Design review of the part shown in the three views and the two pictorial views. Dimensions are in mm from the part's minimum x, y and z. Give positions to 0.01 mm unless a question says otherwise; leave off trailing zeros. Order: outer loops, then holes, each group sorted by start corner. A loop starts at its lowest first (then second) coordinate and runs counter-clockwise, first axis right, second up. Notation, with made-up numbers: (81.25, 63) - (94.25, 63) arc R34 ccw to (94.25, 102) - close; hole circle Ø6 at (-32.5, 68.5). An arc over 180 degrees is marked (long way). Put each result on its own line as item: value.
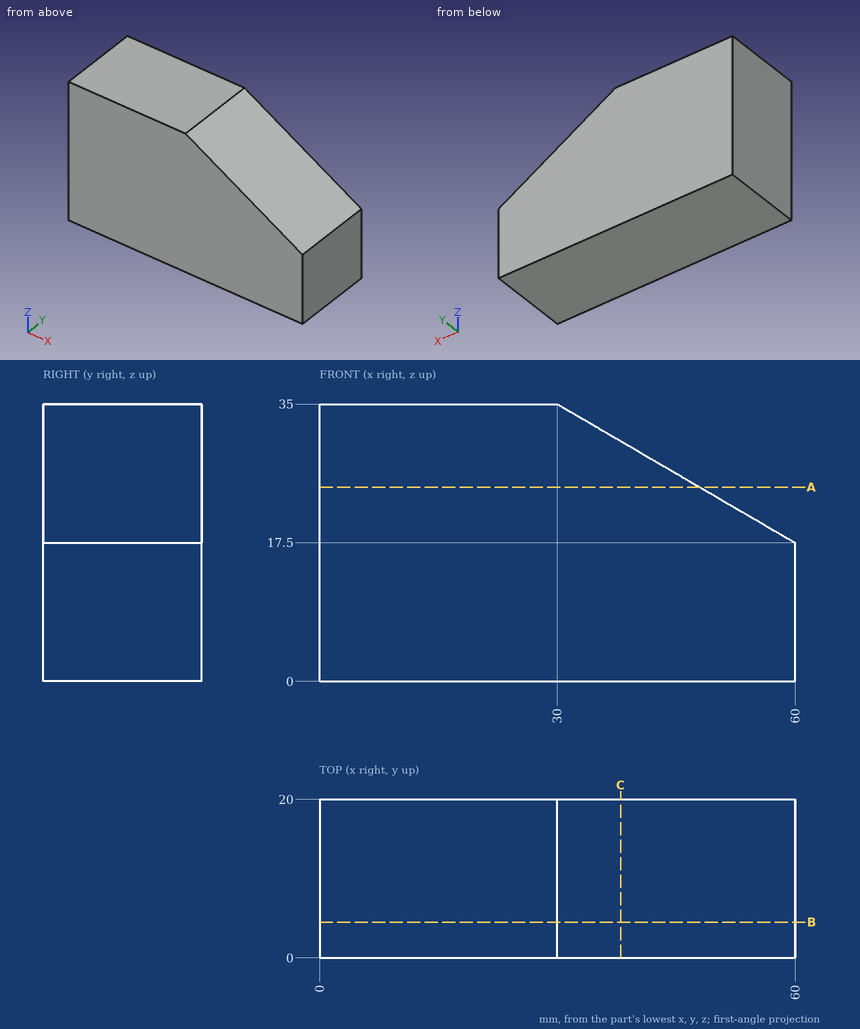
(1) Take a section at C-C, the plane x = 38. Write out the cut boundary in (y, z), then the cut area to 3 significant figures.
The answers:
outline: (0, 0) - (20, 0) - (20, 30.33) - (0, 30.33) - close
area: 607 mm^2
(2) Take a section at B-B, the plane y = 4.5. Write out the cut boundary in (x, z), then the cut area to 3 significant figures.
The answers:
outline: (0, 0) - (60, 0) - (60, 17.5) - (30, 35) - (0, 35) - close
area: 1,840 mm^2
(3) Clearance check with a flat-ended pin moving along its axis: pin 1 Ø4 at (y, z) = (17.5, 20) entering from +X. State where the tip first meets the part, or that it passes through.
The answers:
pin 1: x = 59.14
(4) Wall thickness on L1, parallel to X at y = 4.5, z = 18; L2, parallel to X at y = 5.5, z = 22.5; L3, parallel to Z at x = 43, y = 3: over which ranges is each line inside the solid? List them lowest first.
The answers:
L1: 0 to 59.14
L2: 0 to 51.43
L3: 0 to 27.42
(5) Take a section at A-A, the plane z = 24.5. Write out the cut boundary in (x, y).
The answers:
outline: (0, 0) - (48, 0) - (48, 20) - (0, 20) - close
